Can you work these out from the model? Positions are in its coordinate system, mm. Face numbers are marked on the shaded views. A direction names the side the tool comes from. Round coordinates to 2 decimals unless told otherwise and drop trailing zeros. Write each loop counter-clockwise with the first axis right and the second up, starting at its lowest first coordinate (ties: lowest second). Pieces come first, ordered by that corner, then holes. Notation, with made-up numbers: M 85.25,65.5 L 96.25,65.5 A19 cw 96.25,70.5 Z; hole C -15,63.25 d1. An arc over 180 degrees is marked long. Use one line per item in the form item = value. Start each with the question number.
```python
from build123d import *

# Parameters (mm, degrees)
EXTRUDE_THIN1_DEPTH = 21.59
CUT_EXTRUDE1_REACH  = 39.893
SKETCH2_R           = 1
FILLET1_R           = 2.54


with BuildPart() as part:
    # Sketch1 → Extrude-Thin1 (new body)
    with BuildSketch(Plane(origin=(0, 0, 0), x_dir=(0, 0, -1), z_dir=(1, 0, 0))):
        Polygon((-27.305, -6.35), (-27.305, 0), (27.305, 0), (27.305, -6.35), (29.845, -6.35), (29.845, 2.54), (-29.845, 2.54), (-29.845, -6.35), align=None)
    extrude(amount=EXTRUDE_THIN1_DEPTH)

    # Sketch2 → Cut-Extrude1 (cut, up to next)
    with BuildSketch(Plane(origin=(0, 2.54, 0), x_dir=(1, 0, 0), z_dir=(0, 1, 0)), mode=Mode.PRIVATE) as cut_extrude1_sk1:
        with Locations(Location((3.175, 2.54, 0), (0, 0, 270))):
            Circle(SKETCH2_R)
    cut_extrude1_tool1 = extrude(cut_extrude1_sk1.sketch, amount=-CUT_EXTRUDE1_REACH, mode=Mode.PRIVATE) & part.part
    # Sketch2 → Cut-Extrude1 (cut, up to next)
    with BuildSketch(Plane(origin=(0, 2.54, 0), x_dir=(1, 0, 0), z_dir=(0, 1, 0)), mode=Mode.PRIVATE) as cut_extrude1_sk2:
        with Locations(Location((18.415, 2.54, 0), (0, 0, 270))):
            Circle(SKETCH2_R)
    cut_extrude1_tool2 = extrude(cut_extrude1_sk2.sketch, amount=-CUT_EXTRUDE1_REACH, mode=Mode.PRIVATE) & part.part
    add(cut_extrude1_tool1.solids().sort_by_distance((3.175, 2.54, -2.54))[0], mode=Mode.SUBTRACT)
    add(cut_extrude1_tool2.solids().sort_by_distance((18.415, 2.54, -2.54))[0], mode=Mode.SUBTRACT)

    # Fillet1
    fillet1_edges = [part.edges().sort_by_distance(p)[0] for p in [
        (21.59, -6.35, -28.575),
        (21.59, -6.35, 28.575),
        (0, -6.35, -28.575),
        (0, -6.35, 28.575),
    ]]
    fillet(fillet1_edges, radius=FILLET1_R)


solid = part.part
```
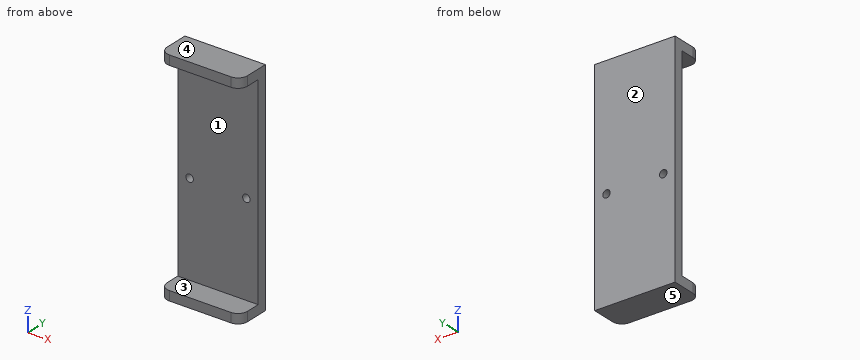
1. If we section it at A-A (z = -2.54): List the corners of the cut face in (x, y) for me (3 decimals), and give its area (3 significant figures).
2. If we section it at D-D (y = -5.25): List the corners of the cut face in (x, z) for me (3 decimals).
3. If we mould it in two halves opening along Z, with no side actions, what happens to the marked faces 3, 4 and 5? For each: pulls with the +Z half, pulls with the -Z half, needs draft (parallel to the pull), parting line crosses it, or undercut.
4. Will this pin go through, and if not, where does the flat tip stop? pin 1 (2 mm diameter, centred on x = 9.5, z = -19, fed in from -Y).
5. Please list where these lines run through material, in increasing order: line 1 along X through (y, z) = (0.95, -2.54) (3 decimals); line 2 along Z through (x, y) = (5.5, -5) (3 decimals); line 3 along Y through (x, z) = (12, 11.5).
6. If we section it at B-B (y = -1.25): List the corners of the cut face in (x, z) for me (3 decimals), and give its area (3 significant figures).
7. Which directions (+Z, -Z, +X, -X, +Y, -Y) give clear straight access to the entire face, cutting with the end or side of a thin tool? Please do the marked faces 1 and 2.
8. If we section it at C-C (x = 8.75): List the corners of the cut face in (y, z) for me (3 decimals).
Model answer:
q1.outline = M 0,0 L 2.175,0 L 2.175,2.54 L 0,2.54 Z; M 4.175,0 L 17.415,0 L 17.415,2.54 L 4.175,2.54 Z; M 19.415,0 L 21.59,0 L 21.59,2.54 L 19.415,2.54 Z
q1.area = 44.7 mm2
q2.outline = M 0.448,-29.845 L 21.142,-29.845 L 21.142,-27.305 L 0.448,-27.305 Z; M 0.448,27.305 L 21.142,27.305 L 21.142,29.845 L 0.448,29.845 Z
q3.face_3 = undercut
q3.face_4 = pulls with the +Z half
q3.face_5 = pulls with the -Z half
q4.pin_1 = 0
q5.line_1 = 0 to 2.175, 4.175 to 17.415, 19.415 to 21.59
q5.line_2 = -29.845 to -27.305, 27.305 to 29.845
q5.line_3 = 0 to 2.54
q6.outline = M 0,-29.845 L 21.59,-29.845 L 21.59,-27.305 L 0,-27.305 Z; M 0,27.305 L 21.59,27.305 L 21.59,29.845 L 0,29.845 Z
q6.area = 110 mm2
q7.face_1 = +X, -X, -Y
q7.face_2 = +Z, -Z, +X, -X, +Y
q8.outline = M -6.35,-29.845 L 2.54,-29.845 L 2.54,29.845 L -6.35,29.845 L -6.35,27.305 L 0,27.305 L 0,-27.305 L -6.35,-27.305 Z
